```python
from build123d import *

# Parameters (mm, degrees)
F0_R     = 15.875
F0_R_2   = 11
F1_DEPTH = 6.35


# Not quite as in the source:
# - a length typed as a fraction of an inch, garbled in the dataset ("3 / 203.2 mm" for 3/8 in), is restored


with BuildPart() as f1:
    # F0 (on Top) → F1 (new body)
    with BuildSketch(Plane.XY):
        Circle(F0_R)
        Circle(F0_R_2, mode=Mode.SUBTRACT)
    extrude(amount=F1_DEPTH)

    # F2 (on Front) → F3 (revolve, cut)
    with BuildSketch(Plane.XZ):
        Polygon((15.875, 0.4327994616), (15.875, 2.7422005384), (13.875, 1.5875), align=None)
        Polygon((15.875, 5.9172005384), (13.875, 4.7625), (15.875, 3.6077994616), align=None)
    revolve(axis=Axis((0, 0, 9.5765832812), (0, 0, 1)), mode=Mode.SUBTRACT)


solid = f1.part
```
Input: part model. Units: mm. Frame: model coordinates. A direction names the side the tool comes from. Round coordinates to 2 decimals unless told otherwise and drop trailing zeros. Answer in a Markdown table with one row per item.
Item 1: Reachability of faces 4 (the conical face through (-3, -13.7, 1.5)), 5 (the cylindrical face through (-3.441, -15.497, 3.169)) from +Z, -Z, +X, -X, +Y, -Y: full face, straight path, thin tool, end or side. Return the list, or none.
Model answer:
| item | result |
|---|---|
| face 4 | none |
| face 5 | +Z, -Z |
Item 2: Pin query (flat end, axial travel): pin 1 (3 mm diameter, centred on x = 5, z = 1, fed in from +Y); pin 2 (1.5 mm diameter, centred on y = -6, z = 1, fed in from -X); pin 3 (2 mm diameter, centred on y = -2.5, z = 4.5, fed in from +X); pin 4 (3 mm diameter, centred on x = -0.5, z = 2.5, fed in from -Y) (3 decimals). Return the tip coordinate at first contact, or that it passes through.
Model answer:
| item | result |
|---|---|
| pin 1 | stops at y = 15.46 |
| pin 2 | stops at x = -14.89 |
| pin 3 | stops at x = 15.74 |
| pin 4 | stops at y = -15.875 |
Item 3: Mould query, pull axis Y, two halves, no side actions, for faces 1 (the cylindrical face through (-2.38, -10.74, 3.13)), 2 (the flat face through (3, 11, 6.35)), 3 (the cylindrical face through (-3.441, -15.497, 6.131)). Classes: released by +Y, released by -Y, zero draft, split by the parting line, or undercut.
Model answer:
| item | result |
|---|---|
| face 1 | undercut |
| face 2 | zero draft |
| face 3 | split by the parting line |
Item 4: Line query: line 1 (Y direction, x = 0, z = 3) (3 decimals); line 2 (Z direction, x = 14.5, y = 4); line 3 (Y direction, x = 0, z = 5). Output: solid intervals per line, ascending.
Model answer:
| item | result |
|---|---|
| line 1 | y = -15.875 to -11, 11 to 15.875 |
| line 2 | z = 0 to 0.91, 2.26 to 4.09, 5.44 to 6.35 |
| line 3 | y = -14.29 to -11, 11 to 14.29 |
